from build123d import *

# Parameters (mm, degrees)
F1_DEPTH = 9.525
F3_DEPTH = 2
F5_D     = 3.3
F5_DEPTH = 12
F5_TIP   = 0.9914200214
F7_DEPTH = 2


with BuildPart() as f1:
    # F0 (on Front) → F1 (new body)
    with BuildSketch(Plane.XZ):
        with BuildLine():
            Line((-17.5, -40), (17.5, -40))
            Line((17.5, -40), (17.5, -15))
            Line((17.5, -15), (9.325, -15))
            Line((9.325, -15), (6, -15))
            Line((6, -15), (6, -30.825))
            ThreePointArc((6, -30.825), (5.0700640303, -33.0700640303), (2.825, -34))
            Line((2.825, -34), (-2.825, -34))
            ThreePointArc((-2.825, -34), (-5.0700640303, -33.0700640303), (-6, -30.825))
            Line((-6, -30.825), (-6, -15))
            Line((-6, -15), (-9.325, -15))
            Line((-9.325, -15), (-17.5, -15))
            Line((-17.5, -15), (-17.5, -40))
        make_face()
        with BuildLine():
            Line((-9.0496408567, -19), (-9.0496408567, -34))
            ThreePointArc((-9.0496408567, -34), (-9.7818739037, -35.767766953), (-11.5496408567, -36.5))
            ThreePointArc((-11.5496408567, -36.5), (-13.3174078096, -35.767766953), (-14.0496408567, -34))
            Line((-14.0496408567, -34), (-14.0496408567, -19))
            ThreePointArc((-14.0496408567, -19), (-13.3174078096, -17.232233047), (-11.5496408567, -16.5))
            ThreePointArc((-11.5496408567, -16.5), (-9.7818739037, -17.232233047), (-9.0496408567, -19))
        make_face(mode=Mode.SUBTRACT)
        with BuildLine():
            ThreePointArc((11.5496408567, -36.5), (9.7818739037, -35.767766953), (9.0496408567, -34))
            Line((9.0496408567, -34), (9.0496408567, -19))
            ThreePointArc((9.0496408567, -19), (9.7818739037, -17.232233047), (11.5496408567, -16.5))
            ThreePointArc((11.5496408567, -16.5), (13.3174078096, -17.232233047), (14.0496408567, -19))
            Line((14.0496408567, -19), (14.0496408567, -34))
            ThreePointArc((14.0496408567, -34), (13.3174078096, -35.767766953), (11.5496408567, -36.5))
        make_face(mode=Mode.SUBTRACT)
        with BuildLine():
            Line((9.325, -15), (17.5, -15))
            Line((17.5, -15), (17.5, 40))
            Line((17.5, 40), (-17.5, 40))
            Line((-17.5, 40), (-17.5, -15))
            Line((-17.5, -15), (-9.325, -15))
            ThreePointArc((-9.325, -15), (-11.5700640303, -14.0700640303), (-12.5, -11.825))
            Line((-12.5, -11.825), (-12.5, 31.825))
            ThreePointArc((-12.5, 31.825), (-11.5700640303, 34.0700640303), (-9.325, 35))
            Line((-9.325, 35), (9.325, 35))
            ThreePointArc((9.325, 35), (11.5700640303, 34.0700640303), (12.5, 31.825))
            Line((12.5, 31.825), (12.5, -11.825))
            ThreePointArc((12.5, -11.825), (11.5700640303, -14.0700640303), (9.325, -15))
        make_face()
    extrude(amount=F1_DEPTH)

    # F2 (on face) → F3 (cut)
    with BuildSketch(Plane.XZ.offset(9.525)):
        with BuildLine():
            Line((-9.325, -15), (-17.5, -15))
            Line((-17.5, -15), (-17.5, -40))
            Line((-17.5, -40), (17.5, -40))
            Line((17.5, -40), (17.5, -15))
            Line((17.5, -15), (9.325, -15))
            Line((9.325, -15), (6, -15))
            Line((6, -15), (6, -30.825))
            ThreePointArc((6, -30.825), (5.0700640303, -33.0700640303), (2.825, -34))
            Line((2.825, -34), (-2.825, -34))
            ThreePointArc((-2.825, -34), (-5.0700640303, -33.0700640303), (-6, -30.825))
            Line((-6, -30.825), (-6, -15))
            Line((-6, -15), (-9.325, -15))
        make_face()
        with BuildLine():
            ThreePointArc((-14.0496408567, -19), (-11.5496408567, -16.5), (-9.0496408567, -19))
            Line((-9.0496408567, -19), (-9.0496408567, -34))
            ThreePointArc((-9.0496408567, -34), (-11.5496408567, -36.5), (-14.0496408567, -34))
            Line((-14.0496408567, -34), (-14.0496408567, -19))
        make_face(mode=Mode.SUBTRACT)
        with BuildLine():
            Line((14.0496408567, -19), (14.0496408567, -34))
            ThreePointArc((14.0496408567, -34), (11.5496408567, -36.5), (9.0496408567, -34))
            Line((9.0496408567, -34), (9.0496408567, -19))
            ThreePointArc((9.0496408567, -19), (11.5496408567, -16.5), (14.0496408567, -19))
        make_face(mode=Mode.SUBTRACT)
    extrude(amount=-F3_DEPTH, mode=Mode.SUBTRACT)

    # F5
    with Locations(Plane.XY.offset(40)):
        with Locations((-13.4, -5.225), (13.4, -5.225)):
            Hole(F5_D / 2, depth=F5_DEPTH)
            with Locations((0, 0, -(F5_DEPTH + F5_TIP / 2))):  # 118° drill point
                Cone(0, F5_D / 2, F5_TIP, mode=Mode.SUBTRACT)

    # F6 (on face) → F7 (cut, through all)
    with BuildSketch(Plane.XZ.offset(9.525)):
        with BuildLine():
            ThreePointArc((-9.325, -15), (-11.5700640303, -14.0700640303), (-12.5, -11.825))
            Line((-12.5, -11.825), (-12.5, -15))
            Line((-12.5, -15), (-9.325, -15))
        make_face()
        with BuildLine():
            Line((12.5, -15), (12.5, -11.825))
            ThreePointArc((12.5, -11.825), (11.5700640303, -14.0700640303), (9.325, -15))
            Line((9.325, -15), (12.5, -15))
        make_face()
    extrude(amount=-F7_DEPTH, mode=Mode.SUBTRACT)


solid = f1.part
Build history of the part. All positions in model axes, mm. A direction names the side the tool comes from. Coordinates: 2 decimals unless noted, no trailing zeros. Write each loop counter-clockwise with the first axis right and the second up, starting at its lowest first coordinate (ties: lowest second). Pieces come first, ordered by that corner, then holes.
(1) 3-axis set-ups, long thin cutter, end or side, ignore diameter. For faces 1 (the cylindrical face through (-14.924, -5.857, 33.916)), 2 (the flat face through (14.05, -4, -26)), 3 (the flat face through (-16, 0, 1)): which of +Z, -Z, +X, -X, +Y, -Y reach the whole face in a straight line?
(2) Cut at B-B on y = -8.25. List the corners of the cut face in (x, z) (3 decimals).
(3) Cut at C-C on x = -4.5. List the corners of the cut face in (y, z) (3 decimals), and give its area (3 significant figures).
(4) Drill centre lines: line 1 (X direction, y = -6, z = -29.5); line 2 (Z direction, x = -1, y = -6.5); line 3 (Y direction, x = -13.4, z = 37.5) (3 decimals). Where is each one in solid material? Low to high.
(5) Mould opens along X. For faces 4 (the flat face through (-12.5, -5, 8)), 5 (the flat face through (17.5, -5, -1)), 6 (the flat face through (0, -4, -40)) say: pulls with the +X half, pulls with the -X half, needs draft (parallel to the pull), parting line crosses it, or undercut.
(6) Cut at D-D on y = -1.5. List the corners of the cut face in (x, z) (3 decimals), and give its area (3 significant figures).
(7) Cut at A-A on z = -2. List the corners of the cut face in (x, y) (3 decimals), and give its area (4 significant figures).
(8) Pin check, flat tips, straight feed: pin 1 Ø2 at (x, y) = (-15, -8) entering from -Z; pin 2 Ø1 at (x, y) = (16, -8.5) entering from -Z; pin 3 Ø2.5 at (x, y) = (-13.4, -5.225) entering from +Z; pin 4 Ø8 at (x, z) = (-5, -14) entering from -Y (3 decimals). Stop position of each tip, or through.
Working result:
1. face 1: +Z
1. face 2: +Y, -Y
1. face 3: +Z, -Z, +X, -X, +Y
2. outline: (-17.5, -15) - (-12.5, -15) - (-12.5, 31.825) arc R3.175 cw to (-9.325, 35) - (9.325, 35) arc R3.175 cw to (12.5, 31.825) - (12.5, -15) - (17.5, -15) - (17.5, 40) - (-17.5, 40) - close
3. outline: (-9.525, 35) - (0, 35) - (0, 40) - (-9.525, 40) - close; (-7.525, -40) - (0, -40) - (0, -33.522) - (-7.525, -33.522) - close
3. area: 96.4 mm2
4. line 1: x = -17.5 to -14.05, -9.05 to -6, 6 to 9.05, 14.05 to 17.5
4. line 2: z = -40 to -34, 35 to 40
4. line 3: y = -9.525 to -6.875, -3.575 to 0
5. face 4: undercut
5. face 5: pulls with the +X half
5. face 6: needs draft
6. outline: (-17.5, -40) - (17.5, -40) - (17.5, 40) - (-17.5, 40) - close; hole (-14.05, -34) arc R2.5 ccw to (-9.05, -34) - (-9.05, -19) arc R2.5 ccw to (-14.05, -19) - close; hole (-12.5, -11.825) arc R3.175 ccw to (-9.325, -15) - (-6, -15) - (-6, -30.825) arc R3.175 ccw to (-2.825, -34) - (2.825, -34) arc R3.175 ccw to (6, -30.825) - (6, -15) - (9.325, -15) arc R3.175 ccw to (12.5, -11.825) - (12.5, 31.825) arc R3.175 ccw to (9.325, 35) - (-9.325, 35) arc R3.175 ccw to (-12.5, 31.825) - close; hole (9.05, -34) arc R2.5 ccw to (14.05, -34) - (14.05, -19) arc R2.5 ccw to (9.05, -19) - close
6. area: 1,150 mm2
7. outline: (-17.5, -9.525) - (-12.5, -9.525) - (-12.5, 0) - (-17.5, 0) - close; (12.5, -9.525) - (17.5, -9.525) - (17.5, 0) - (12.5, 0) - close
7. area: 95.25 mm2
8. pin 1: stops at z = -40
8. pin 2: stops at z = -15
8. pin 3: stops at z = 27.76
8. pin 4: stops at y = -7.525
